Work out the finished part from the listing and answer in its coordinate system (mm). A direction names the side the tool comes from. Round coordinates to 2 decimals unless told otherwise and drop trailing zeros. Loops run counter-clockwise (first coordinate to the right, second up) from the corner with the lowest first, then second, coordinate; pieces in that order, holes last. Notation, with made-up numbers: (66, 75.25) -> (106, 75.25) arc R33 cw to (106, 109.25) -> close; hole circle Ø8 at (20, 36). An arc over 180 degrees is marked (long way). Use CSV: the item, a comma, the result in double quotes. Start each with the question number.
from build123d import *

# Parameters (mm, degrees)
SKETCH2_W           = 64
SKETCH2_H           = 96
BOSS_EXTRUDE1_DEPTH = 16
SKETCH3_W           = 64
SKETCH3_H           = 16
BOSS_EXTRUDE3_DEPTH = 48
FILLET3_R           = 48
SKETCH5_W           = 40
SKETCH5_H           = 40
BOSS_EXTRUDE4_DEPTH = 28
SKETCH6_R           = 12
CUT_EXTRUDE1_DEPTH  = 63
SKETCH7_W           = 12.002152701
SKETCH7_H           = 40
BOSS_EXTRUDE6_DEPTH = 28
CUT_EXTRUDE2_DEPTH  = 30
CUT_EXTRUDE3_DEPTH  = 17


with BuildPart() as part:
    # Sketch2 → Boss-Extrude1 (new body)
    with BuildSketch(Plane(origin=(0, 0, 0), x_dir=(1, 0, 0), z_dir=(0, 1, 0))):
        Rectangle(SKETCH2_W, SKETCH2_H)
    extrude(amount=BOSS_EXTRUDE1_DEPTH)

    # Sketch3 → Boss-Extrude3 (add)
    with BuildSketch(Plane(origin=(0, 16, 0), x_dir=(1, 0, 0), z_dir=(0, 1, 0))):
        with Locations((0, 40)):
            Rectangle(SKETCH3_W, SKETCH3_H)
    extrude(amount=BOSS_EXTRUDE3_DEPTH)

    # Fillet3
    fillet3_edges = [part.edges().sort_by_distance(p)[0] for p in [
        (-32, 64, -40),
    ]]
    fillet(fillet3_edges, radius=FILLET3_R)

    # Sketch5 → Boss-Extrude4 (add)
    with BuildSketch(Plane(origin=(0, 16, 0), x_dir=(1, 0, 0), z_dir=(0, 1, 0))):
        with Locations((12, 12)):
            Rectangle(SKETCH5_W, SKETCH5_H)
    extrude(amount=BOSS_EXTRUDE4_DEPTH)

    # Sketch6 → Cut-Extrude1 (cut)
    with BuildSketch(Plane.ZY.offset(8)):
        with Locations((-12, 44)):
            Circle(SKETCH6_R)
    extrude(amount=-CUT_EXTRUDE1_DEPTH, mode=Mode.SUBTRACT)

    # Sketch7 → Boss-Extrude6 (add)
    with BuildSketch(Plane(origin=(0, 16, 0), x_dir=(1, 0, 0), z_dir=(0, 1, 0))):
        with Locations((25.99892365, -28)):
            Rectangle(SKETCH7_W, SKETCH7_H)
    extrude(amount=BOSS_EXTRUDE6_DEPTH)

    # Sketch9 → Cut-Extrude2 (cut)
    with BuildSketch(Plane.ZY.offset(-19.997847299)):
        Polygon((8, 44), (48, 16), (48, 44), align=None)
    extrude(amount=-CUT_EXTRUDE2_DEPTH, mode=Mode.SUBTRACT)

    # Sketch10 → Cut-Extrude3 (cut, through all)
    with BuildSketch(Plane(origin=(0, 16, 0), x_dir=(1, 0, 0), z_dir=(0, 1, 0))):
        with BuildLine():
            Line((-16, -48), (-16, -28))
            ThreePointArc((-16, -28), (-8, -20), (0, -28))
            Line((0, -28), (0, -48))
            ThreePointArc((0, -48), (-8, -56), (-16, -48))
        make_face()
    extrude(amount=-CUT_EXTRUDE3_DEPTH, mode=Mode.SUBTRACT)


solid = part.part
Q1. Each of these flat-tipped pins is pushed along its axis until it touches: pin 1 (10 mm diameter, centred on y = 42, z = 26.5, fed in from +X); pin 2 (24 mm diameter, centred on x = -8.5, y = 48.5, fed in from +Z); pin 3 (8 mm diameter, centred on x = -17.5, z = -31.5, fed in from +Y); pin 4 (22.5 mm diameter, centred on y = 34, z = 20.5, fed in from -X). Where does it stop, or does it pass through?
Q2. Straight lines are drawn through the part: line 1 (X direction, y = 6.5, z = 23) (3 decimals); line 2 (Y direction, x = -21, z = 42); line 3 (Z direction, x = -8, y = 6.5). For each, find the intervals that lie inside material, in ascending order. Write a range as from..to.
Q3. Which of the six approach directions +Z, -Z, +X, -X, +Y, -Y give full straight-line access (tool end or side, diameter ignored) to faces 1 (the flat face through (-24, 8, 48)), 2 (the flat face through (-8, 27, -12)), 3 (the flat face through (24, 64, -40)), 4 (the flat face through (12, 44, 4)), 5 (the flat face through (-16, 8, 38))?
Q4. Section D-D, the plane y = 8.5 is taken. Write down the section's boundary in (x, z), and give its area (3 significant figures).
Q5. For a pull along X with two mould halves and no side action, classify faces 6 (the flat face through (12, 44, -28)), 7 (the flat face through (32, 17, -10)), 8 (the flat face through (0, 8, 38)) as pulls with the +X half, pulls with the -X half, needs draft (parallel to the pull), parting line crosses it, or undercut.
Q6. Section A-A, the plane y = 40 is taken. Write down the section's boundary in (x, z), and give its area (3 significant figures).
Q7. Section C-C, the plane x = 22 is taken. Write down the section's boundary in (y, z), and give its area (3 significant figures).
Q8. Section B-B, the plane z = 29.5 is taken. Write down the section's boundary in (x, y), and give its area (3 significant figures).
Report:
1,pin 1,"passes through"
1,pin 2,"stops at z = 8"
1,pin 3,"stops at y = 53.84"
1,pin 4,"stops at x = 20"
2,line 1,"x = -32..-14.245, -1.755..32"
2,line 2,"y = 0..16"
2,line 3,"z = -48..20"
3,face 1,"+Z, +X, -X, +Y, -Y"
3,face 2,"+Z, -X, +Y"
3,face 3,"+Z, -Z, +X, -X, +Y"
3,face 4,"+Z, +X, -X, +Y"
3,face 5,"+Z, +Y, -Y"
4,outline,"(-32, -48) -> (32, -48) -> (32, 48) -> (0, 48) -> (0, 28) arc R8 cw to (-16, 28) -> (-16, 48) -> (-32, 48) -> close"
4,area,"5,720 mm²"
5,face 6,"needs draft"
5,face 7,"pulls with the +X half"
5,face 8,"undercut"
6,outline,"(-25.57, -48) -> (32, -48) -> (32, -23.31) -> (-8, -23.31) -> (-8, -32) -> (-25.57, -32) -> close; (-8, -0.69) -> (32, -0.69) -> (32, 13.71) -> (20, 13.71) -> (20, 8) -> (-8, 8) -> close"
6,area,"1,680 mm²"
7,outline,"(0, -48) -> (64, -48) -> (64, -32) -> (44, -32) -> (44, -24) arc R12 cw to (44, 0) -> (44, 8) -> (16, 48) -> (0, 48) -> close"
7,area,"3,760 mm²"
8,outline,"(-32, 0) -> (-16, 0) -> (-16, 16) -> (-32, 16) -> close; (0, 0) -> (32, 0) -> (32, 28.95) -> (20, 28.95) -> (20, 16) -> (0, 16) -> close"
8,area,"923 mm²"
